Build history of the part. All positions in model axes, mm. A direction names the side the tool comes from. Coordinates: 2 decimals unless noted, no trailing zeros. Write each loop counter-clockwise with the first axis right and the second up, starting at its lowest first coordinate (ties: lowest second). Pieces come first, ordered by that corner, then holes. Notation, with made-up numbers: M 32.5,-14 L 80.5,-14 A12 cw 80.5,-5 Z; hole C 64.25,30 d6. An arc over 180 degrees is marked long. Use CSV: the item, a comma, the result in double quotes. Start each with the question number.
```python
from build123d import *

# Parameters (mm, degrees)
F0_W     = 40
F0_H     = 38
F0_R     = 10
F1_DEPTH = 10
F4_D     = 3.5
F2_R     = 15
F2_R_2   = 10
F5_DEPTH = 50
F6_R     = 1.5
F7_DEPTH = 25
F8_R     = 1.99999


# Not quite as in the source:
# - a fillet or chamfer that OpenCascade refuses, or shapes differently, is made with other operations: its cross-section is extruded or revolved along the edge and cut away or added
# - a fillet or chamfer is up to 0.001 mm smaller than in the source, because OpenCascade refuses the exact size


with BuildPart() as f1:
    # F0 (on Top) → F1 (new body)
    with BuildSketch(Plane.XY):
        Rectangle(F0_W, F0_H)
        Circle(F0_R, mode=Mode.SUBTRACT)
    extrude(amount=F1_DEPTH)

    # F4 (through all)
    with Locations(Plane.XY.offset(10)):
        with Locations((-14, 13), (-14, -13), (14, -13), (14, 13)):
            Hole(F4_D / 2)

    # F2 (on face) → F5 (join)
    with BuildSketch(Plane.XY.offset(10)):
        Circle(F2_R)
        Circle(F2_R_2, mode=Mode.SUBTRACT)
    extrude(amount=F5_DEPTH)

    # F6 (on Front) → F7 (cut)
    with BuildSketch(Plane.XZ):
        with Locations((0, 35)):
            Circle(F6_R)
    extrude(amount=F7_DEPTH, mode=Mode.SUBTRACT)

    # F8 (radius 2 in the source; OpenCascade refuses exactly that, so slightly less here)
    f8_edges = [f1.edges().sort_by_distance(p)[0] for p in [
        (-15, 0, 10),
        (20, 0, 10),
        (0, -19, 10),
        (-20, 0, 10),
        (0, 19, 10),
        (20, 19, 5),
        (-20, -19, 5),
        (20, -19, 5),
        (-15, 0, 60),
        (-20, 19, 5),
    ]]
    fillet(f8_edges, radius=F8_R)

    # F9: chamfer of 4 on 1 edges, made by hand

    # F9_s1 → F9_t2 (revolve, cut)
    with BuildSketch(Plane.XZ):
        Polygon((10, 56), (14, 60), (10, 60), align=None)
    revolve(axis=Axis((0, 0, 60), (0, 0, 1)), mode=Mode.SUBTRACT)


solid = f1.part
```
1. Slice it at C-C (z = 22.5). List the corners of the cut face in (x, y), and give its area (3 significant figures).
2. Flat gauge pins, fed straight in: pin 1 (2 mm diameter, centred on x = -4.5, z = 47, fed in from +Y); pin 2 (1.5 mm diameter, centred on x = 6, z = 26.5, fed in from +Y); pin 3 (10 mm diameter, centred on y = 3, z = 48.5, fed in from +X). Where does each tip first touch, or does it go through?
3. Drill centre lines: line 1 along Y through (x, z) = (-14, 3); line 2 along Y through (x, z) = (0, 26.5); line 3 along Z through (x, y) = (16.5, 14). Where is each one in solid material? Low to high. Write a range as from..to.
4. 3-axis set-ups, long thin cutter, end or side, ignore diameter. For faces 4 (the flat face through (0, 19, 4)), 5 (the cylindrical face through (-0.325, -12.407, 33.536)), 6 (the cylindrical face through (-14.985, 0.66, 34.678)): which of +Z, -Z, +X, -X, +Y, -Y reach the whole face in a straight line?
5. Pull direction X, two halves, no side cores. Call faces 1 (the cylindrical face through (14.228, -11.265, 4.93)), 2 (the cylindrical face through (-19.4, 0.24, 9.43)), 3 (the cylindrical face through (0.25, -18.4, 9.43)): pulls with the +X half, pulls with the -X half, needs draft (parallel to the pull), parting line crosses it, or undercut.
6. Slice it at A-A (x = 0). Count the separate pieces of the cut face and the enclosed holes in it, and give its area (3 significant figures).
7. Slice it at B-B (y = 0). List the corners of the cut face in (x, z), and give its area (3 significant figures).
Established:
1,outline,"C 0,0 d30; hole C 0,0 d20"
1,area,"393 mm2"
2,pin 1,"stops at y = 14.59"
2,pin 2,"stops at y = 14.05"
2,pin 3,"stops at x = 15"
3,line 1,"y = -19..-14.75, -11.25..11.25, 14.75..19"
3,line 2,"y = -15..-10, 10..15"
3,line 3,"z = 0..10"
4,face 4,"+Z, -Z, +X, -X, +Y"
4,face 5,"-Y"
4,face 6,"+Z"
5,face 1,"undercut"
5,face 2,"pulls with the -X half"
5,face 3,"needs draft"
6,separate pieces,"3"
6,enclosed holes,"0"
6,area,"647 mm2"
7,outline,"M -20,0 L -10,0 L -10,56 L -13.82,59.82 A2 ccw -15,58 L -15,12 A2 cw -17,10 L -18,10 A2 ccw -20,8 Z; M 10,0 L 20,0 L 20,8 A2 ccw 18,10 L 17,10 A2 cw 15,12 L 15,58 A2 ccw 13.82,59.82 L 10,56 Z"
7,area,"682 mm2"
